from build123d import *

# Parameters (mm, degrees)
SM_START               = -161.965
SM_BASE_FLANGE_1_DEPTH = 323.93
FILLET_3_R             = 10
FILLET_4_R             = 10
FILLET_5_R             = 10
FILLET_6_R             = 10
FILLET_7_R             = 10


# Read off the part's stored shape, not the designer's step: 基体-法兰1
with BuildPart() as part:
    # 基体-法兰1 outline → 基体-法兰1 (new body)
    with BuildSketch(Plane(origin=(0, 0, 0), x_dir=(0, 0, -1), z_dir=(1, 0, 0)).offset(SM_START)):
        Polygon((-4.503882243, 0), (0, 0), (0, 49.038822429), (-18.519411214, 49.038822429), (-18.519411214, 63.558233643), (0, 63.558233643), (0, 112.597056072), (-4.503882243, 112.597056072), (-4.503882243, 67.558233643), (-22.519411214, 67.558233643), (-22.519411214, 45.038822429), (-4.503882243, 45.038822429), align=None)
    extrude(amount=SM_BASE_FLANGE_1_DEPTH)

    # 圆角3
    fillet_3_edges = [part.edges().sort_by_distance(p)[0] for p in [
        (0, 45.038822429, 22.519411214),
        (0, 67.558233643, 22.519411214),
    ]]
    fillet(fillet_3_edges, radius=FILLET_3_R)

    # 圆角4
    # the kernel refuses this fillet: 10 mm, written as the material it adds along each edge
    with BuildSketch(Plane(origin=(-161.965, 49.038822429, 18.519411214), x_dir=(0, 1, 0), z_dir=(1, 0, 0)), Plane(origin=(-161.965, 63.558233643, 18.519411214), x_dir=(0, 0, -1), z_dir=(1, 0, 0))) as fillet_4_piece_1:
        with BuildLine():
            CenterArc((FILLET_4_R, -FILLET_4_R), FILLET_4_R, 90, 90)
            Line((0, -FILLET_4_R), (0, 0))
            Line((0, 0), (FILLET_4_R, 0))
        make_face()
    extrude(amount=323.93)

    # 圆角5
    fillet_5_edges = [part.edges().sort_by_distance(p)[0] for p in [
        (0, 63.558233643, 0),
        (0, 49.038822429, 0),
    ]]
    fillet(fillet_5_edges, radius=FILLET_5_R)

    # 圆角6
    fillet_6_edges = [part.edges().sort_by_distance(p)[0] for p in [
        (0, 45.038822429, 4.503882243),
    ]]
    fillet(fillet_6_edges, radius=FILLET_6_R)

    # 圆角7
    fillet_7_edges = [part.edges().sort_by_distance(p)[0] for p in [
        (0, 67.558233643, 4.503882243),
    ]]
    fillet(fillet_7_edges, radius=FILLET_7_R)


solid = part.part
Model file for the job. Use its own axes, mm. A direction names the side the tool comes from. Coordinates: 2 decimals unless noted, no trailing zeros. Write each loop counter-clockwise with the first axis right and the second up, starting at its lowest first coordinate (ties: lowest second). Pieces come first, ordered by that corner, then holes. Notation, with made-up numbers: (53, 16.5) - (101, 16.5) arc R24 cw to (101, 55.5) - close; hole circle Ø8 at (58.5, 44.25). An arc over 180 degrees is marked (long way). Write each question's results on one line, items separated by ' | '. Start each with the question number.
1) 3-axis set-ups, long thin cutter, end or side, ignore diameter. For faces 1 (the face through (-2.27, 51.34, 14.9)), 2 (the face through (-2, 19, 0)), 3 (the face through (-2, 95, 4.504)): which of +Z, -Z, +X, -X, +Y, -Y reach the whole face in a straight line?
2) Probe line 1 along Y through (x, z) = (130, 2); line 2 along Z through (x, y) = (-77.5, 102.5); line 3 along Y through (x, z) = (26.5, 2.5). List the from-to ranges inside material, lowest first. Write a range as from..to.
3) Mould opens along Y. For faces 4 (the face through (2.27, 64.35, 19.86)), 5 (the face through (-2, 18, 4.504)), 6 (the face through (-2.268, 61.365, 14.769)) say: pulls with the +Y half, pulls with the -Y half, needs draft (parallel to the pull), parting line crosses it, or undercut.
4) Cut at B-B (y = 60.5). Write the cut outline in (x, z) (3 decimals).
5) Cut at A-A (y = 16.5). Write the cut outline in (x, z) (3 decimals), then the cut area to 3 significant figures.
6) Flat gauge pins, fed straight in: P1, Ø1, axis at x = -17.5, y = 57, coming from the -Z side; P2, Ø10.5, axis at x = 66, y = 10, coming from the +Z side; P3, Ø6, axis at y = 70.5, z = 12.5, coming from the -X side (3 decimals); P4, Ø5, axis at x = -107.5, z = 8, coming from the -Y side. Where does each tip first touch, or does it go through?
Returned:
1) face 1: -Z, +X, -X | face 2: -Z, +X, -X, +Y, -Y | face 3: +Z, +X, -X, +Y
2) line 1: 0..45.09, 67.5..112.6 | line 2: 0..4.5 | line 3: 0..45.71, 66.89..112.6
3) face 4: pulls with the +Y half | face 5: needs draft | face 6: undercut
4) outline: (-161.965, 15.717) - (161.965, 15.717) - (161.965, 22.077) - (-161.965, 22.077) - close
5) outline: (-161.965, 0) - (161.965, 0) - (161.965, 4.504) - (-161.965, 4.504) - close | area: 1,460 mm^2
6) P1: z = 17.71 | P2: z = 4.5 | P3: x = -161.965 | P4: y = 39.49
